```python
from build123d import *

# Parameters (mm, degrees)
SKETCH_1_W                   = 8
SKETCH_1_H                   = 4.984423676
EXTRUDE_1_DEPTH              = 20
SKETCH_2_R                   = 2
CUT_EXTRUDE_1_DEPTH          = 20
SKETCH_2_3_R                 = 2
CUT_EXTRUDE_2_DEPTH          = 20
SKETCH_2_4_R                 = 7.5
EXTRUDE_2_DEPTH              = 1
SKETCH_2_5_R                 = 6
EXTRUDE_3_DEPTH              = 2
SKETCH_2_6_R                 = 3
EXTRUDE_4_DEPTH              = 5
HOLE_WIZARD_M3_2_D           = 2.5
HOLE_WIZARD_M3_2_DEPTH       = 2
HOLE_WIZARD_M3_2_CSINK_D     = 2.55
HOLE_WIZARD_M3_2_CSINK_ANGLE = 90
FILLET_1_R                   = 1
FILLET_2_R                   = 1


with BuildPart() as part:
    # Sketch 1 → Extrude 1 (new body)
    with BuildSketch(Plane.XY):
        Polygon((40, 39), (20, 39), (20, 0), (40, 0), (40, 26.015576324), (40, 31), align=None)
        Polygon((20, 0), (20, 39), (0, 39), (0, 31), (0, 26.015576324), (0, 0), align=None)
        with Locations((44, 28.507788162)):
            Rectangle(SKETCH_1_W, SKETCH_1_H)
        with Locations((-4, 28.507788162)):
            Rectangle(SKETCH_1_W, SKETCH_1_H)
    extrude(amount=EXTRUDE_1_DEPTH)

    # Sketch 2 → Cut-Extrude 1 (cut)
    with BuildSketch(Plane(origin=(0, 39, 0), x_dir=(1, 0, 0), z_dir=(0, 1, 0))):
        with Locations(Location((-4, -15, 0), (0, 0, 90))):
            Circle(SKETCH_2_R)
    extrude(amount=-CUT_EXTRUDE_1_DEPTH, mode=Mode.SUBTRACT)

    # Sketch 2_3 → Cut-Extrude 2 (cut)
    with BuildSketch(Plane(origin=(0, 39, 0), x_dir=(1, 0, 0), z_dir=(0, 1, 0))):
        with Locations(Location((-4, -5, 0), (0, 0, 90))):
            Circle(SKETCH_2_3_R)
        with Locations(Location((44, -5, 0), (0, 0, 270))):
            Circle(SKETCH_2_3_R)
        with Locations(Location((44, -15, 0), (0, 0, 270))):
            Circle(SKETCH_2_3_R)
    extrude(amount=-CUT_EXTRUDE_2_DEPTH, mode=Mode.SUBTRACT)

    # Sketch 2_4 → Extrude 2 (add)
    with BuildSketch(Plane(origin=(0, 39, 0), x_dir=(1, 0, 0), z_dir=(0, 1, 0))):
        with Locations(Location((10, -10, 0), (0, 0, 270))):
            Circle(SKETCH_2_4_R)
    extrude(amount=EXTRUDE_2_DEPTH)

    # Sketch 2_5 → Extrude 3 (add)
    with BuildSketch(Plane(origin=(0, 39, 0), x_dir=(1, 0, 0), z_dir=(0, 1, 0))):
        with Locations(Location((10, -10, 0), (0, 0, 270))):
            Circle(SKETCH_2_5_R)
    extrude(amount=EXTRUDE_3_DEPTH)

    # Sketch 2_6 → Extrude 4 (add)
    with BuildSketch(Plane(origin=(0, 39, 0), x_dir=(1, 0, 0), z_dir=(0, 1, 0))):
        with Locations(Location((10, -10, 0), (0, 0, 270))):
            Circle(SKETCH_2_6_R)
    extrude(amount=EXTRUDE_4_DEPTH)

    # Hole Wizard M3 _2
    with Locations(Plane(origin=(10, 44, 10), x_dir=(0, 0, 1), z_dir=(0, 1, 0))):
        with Locations((0, 0)):
            CounterSinkHole(HOLE_WIZARD_M3_2_D / 2, HOLE_WIZARD_M3_2_CSINK_D / 2, depth=HOLE_WIZARD_M3_2_DEPTH, counter_sink_angle=HOLE_WIZARD_M3_2_CSINK_ANGLE)

    # Fillet 1
    fillet_1_edges = [part.edges().sort_by_distance(p)[0] for p in [
        (-8, 28.507788162, 20),
    ]]
    fillet(fillet_1_edges, radius=FILLET_1_R)

    # Fillet 2
    fillet_2_edges = [part.edges().sort_by_distance(p)[0] for p in [
        (48, 28.507788162, 0),
        (48, 28.507788162, 20),
        (-8, 28.507788162, 0),
    ]]
    fillet(fillet_2_edges, radius=FILLET_2_R)


solid = part.part
```
Work out the finished part from the listing and answer in its coordinate system (mm). A direction names the side the tool comes from. Give positions to 0.01 mm unless a question says otherwise; leave off trailing zeros. Order: outer loops, then holes, each group sorted by start corner. A loop starts at its lowest first (then second) coordinate and runs counter-clockwise, first axis right, second up. Notation, with made-up numbers: (-40, 74) -> (-34, 74) arc R32 cw to (-34, 106) -> close; hole circle Ø10 at (-28, -9.5). An arc over 180 degrees is marked (long way). Answer as CSV lines item,"result". Start each with the question number.
(1) Each of these flat-tipped pins is pushed along its axis until it touches: pin 1 Ø2 at (y, z) = (9.5, 2.5) entering from -X; pin 2 Ø10 at (y, z) = (16, 10.5) entering from +X; pin 3 Ø6.5 at (x, z) = (-3, 7.5) entering from +Y. Where does it stop, or does it pass through?
(2) Consider line 1 along X through (y, z) = (28.4, 15); line 2 along X through (y, z) = (43.45, 10). Determine where each line is inside the solid, lowest interval first.
(3) Which of the six approach directions +Z, -Z, +X, -X, +Y, -Y give full straight-line access (tool end or side, diameter ignored) to faces 4 (the flat face through (40, 35, 10)), 5 (the flat face through (-4, 31, 10)), 6 (the cylindrical face through (4.143, 40.493, 8.699))?
(4) Section A-A, the plane y = 30 is taken. Write down the section's boundary in (x, z).
(5) Section B-B, the plane x = -4 is taken. Write down the section's boundary in (y, z), plus the area to 3 significant figures.
(6) Section D-D, the plane z = 6 is taken. Write down the section's boundary in (x, y).
(7) For a pull along X with two mould halves and no side action, classify faces 1 (the flat face through (10, 42, 10)), 2 (the cylindrical face through (2.68, 39.49, 8.37)), 3 (the flat face through (44, 31, 10)) as released by +X, released by -X, zero draft, split by the parting line, or undercut.
Entries:
1,pin 1,"x = 0"
1,pin 2,"x = 40"
1,pin 3,"y = 39"
2,line 1,"-8 to -6, -2 to 42, 46 to 48"
2,line 2,"7 to 8.75, 11.25 to 13"
3,face 4,"+Z, -Z, +X, +Y"
3,face 5,"+Z, -Z, -X, +Y"
3,face 6,"+Y"
4,outline,"(-8, 1) arc R1 ccw to (-7, 0) -> (47, 0) arc R1 ccw to (48, 1) -> (48, 19) arc R1 ccw to (47, 20) -> (-7, 20) arc R1 ccw to (-8, 19) -> close; hole circle Ø4 at (-4, 5); hole circle Ø4 at (-4, 15); hole circle Ø4 at (44, 5); hole circle Ø4 at (44, 15)"
5,outline,"(26.02, 0) -> (31, 0) -> (31, 3) -> (26.02, 3) -> close; (26.02, 7) -> (31, 7) -> (31, 13) -> (26.02, 13) -> close; (26.02, 17) -> (31, 17) -> (31, 20) -> (26.02, 20) -> close"
5,area,"59.8 mm²"
6,outline,"(-8, 26.02) -> (-5.73, 26.02) -> (-5.73, 31) -> (-8, 31) -> close; (-2.27, 26.02) -> (0, 26.02) -> (0, 0) -> (40, 0) -> (40, 26.02) -> (42.27, 26.02) -> (42.27, 31) -> (40, 31) -> (40, 39) -> (16.34, 39) -> (16.34, 40) -> (14.47, 40) -> (14.47, 41) -> (5.53, 41) -> (5.53, 40) -> (3.66, 40) -> (3.66, 39) -> (0, 39) -> (0, 31) -> (-2.27, 31) -> close; (45.73, 26.02) -> (48, 26.02) -> (48, 31) -> (45.73, 31) -> close"
7,face 1,"undercut"
7,face 2,"split by the parting line"
7,face 3,"zero draft"
